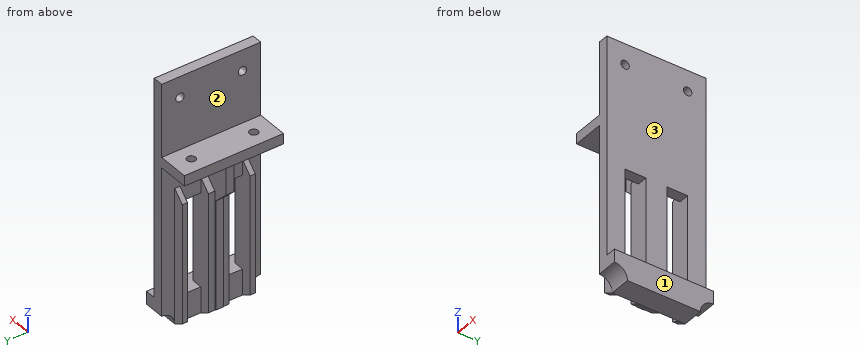
from build123d import *

# Parameters (mm, degrees)
F0_W      = 25.4
F0_H      = 228.6
F1_DEPTH  = 120.65
F2_DEPTH  = 76.2
F3_DEPTH  = 25.4
F4_R      = 10.31875
F5_DEPTH  = 101.601
F7_DEPTH  = 127.001
F9_DEPTH  = 88.9
F10_DEPTH = 76.2
F11_DEPTH = 25.4
F12_DEPTH = 9.525
F13_R     = 10.31875
F14_DEPTH = 419.031


with BuildPart() as f1:
    # F0 (on Front) → F1 (new body, symmetric)
    with BuildSketch(Plane.XZ):
        with Locations((-12.7, 114.3)):
            Rectangle(F0_W, F0_H)
        Polygon((-25.4, 228.6), (0, 228.6), (0, 533.6), (-25.4, 533.6), (-25.4, 355.73), (-101.6, 355.73), (-101.6, 330.33), (-25.4, 330.33), align=None)
        Polygon((25.4, 0), (0, 0), (-25.4, 0), (-25.4, -63.3), (25.4, -63.3), align=None)
    extrude(amount=F1_DEPTH, both=True)

    # F0 (on Front) → F2 (cut, symmetric)
    with BuildSketch(Plane.XZ):
        with Locations((-12.7, 114.3)):
            Rectangle(F0_W, F0_H)
    extrude(amount=F2_DEPTH, both=True, mode=Mode.SUBTRACT)

    # F0 (on Front) → F3 (join, symmetric)
    with BuildSketch(Plane.XZ):
        with Locations((-12.7, 114.3)):
            Rectangle(F0_W, F0_H)
    extrude(amount=F3_DEPTH, both=True)

    # F4 (on face) → F5 (cut, through all)
    with BuildSketch(Plane.YZ):
        with Locations((-76.2, 482.6)):
            Circle(F4_R)
        with Locations((76.2, 482.6)):
            Circle(F4_R)
    extrude(amount=-F5_DEPTH, mode=Mode.SUBTRACT)

    # F6 (on face) → F7 (cut, through all)
    with BuildSketch(Plane.YZ.offset(25.4)):
        with BuildLine():
            Line((-120.65, -63.3), (-88.9, -63.3))
            ThreePointArc((-88.9, -63.3), (-98.1993596973, -40.8493596973), (-120.65, -31.55))
            Line((-120.65, -31.55), (-120.65, -63.3))
        make_face()
        with BuildLine():
            ThreePointArc((120.65, -31.55), (98.1993596973, -40.8493596973), (88.9, -63.3))
            Line((88.9, -63.3), (120.65, -63.3))
            Line((120.65, -63.3), (120.65, -31.55))
        make_face()
    extrude(amount=-F7_DEPTH, mode=Mode.SUBTRACT)

    # F8 (on Front) → F9 (join, symmetric)
    with BuildSketch(Plane.XZ):
        Polygon((-50.8, -48.6353031626), (-25.4, -63.3), (-25.4, 266.83), (-50.8, 241.43), (-50.8, 216.03), align=None)
    extrude(amount=F9_DEPTH, both=True)

    # F8 (on Front) → F10 (cut, symmetric)
    with BuildSketch(Plane.XZ):
        Polygon((-50.8, -48.6353031626), (-25.4, -63.3), (-25.4, 266.83), (-50.8, 241.43), (-50.8, 216.03), align=None)
    extrude(amount=F10_DEPTH, both=True, mode=Mode.SUBTRACT)

    # F8 (on Front) → F11 (join, symmetric)
    with BuildSketch(Plane.XZ):
        Polygon((-50.8, -48.6353031626), (-25.4, -63.3), (-25.4, 266.83), (-50.8, 241.43), (-50.8, 216.03), align=None)
    extrude(amount=F11_DEPTH, both=True)

    # F8 (on Front) → F12 (join, symmetric)
    with BuildSketch(Plane.XZ):
        Polygon((-50.8, 241.43), (-25.4, 266.83), (-25.4, 330.33), (-88.9, 330.33), (-88.9, 254.13), (-53.975, 219.205), (-50.8, 216.03), align=None)
        Polygon((-53.975, -46.8022160579), (-50.8, -48.6353031626), (-50.8, 216.03), (-53.975, 219.205), align=None)
    extrude(amount=F12_DEPTH, both=True)

    # F13 (on face) → F14 (cut, through all)
    with BuildSketch(Plane.XY.offset(355.73)):
        with Locations((-63.5, 76.2)):
            Circle(F13_R)
        with Locations((-63.5, -76.2)):
            Circle(F13_R)
    extrude(amount=-F14_DEPTH, mode=Mode.SUBTRACT)


solid = f1.part
Could you check a few things on this model? Use its own coordinates, in mm. Face numbers are marked on the shaded views. A direction names the side the tool comes from. Round coordinates to 2 decimals unless told otherwise and drop trailing zeros. Write each loop counter-clockwise with the first axis right and the second up, starting at its lowest first coordinate (ties: lowest second). Pieces come first, ordered by that corner, then holes. Notation, with made-up numbers: (11.25, 54) - (44.25, 54) arc R24 cw to (44.25, 80) - close; hole circle Ø3 at (71, 5). An arc over 180 degrees is marked (long way). Use a Markdown table: item, result.
Q1. Please list where these lines run through material, in increasing order: L1, parallel to Y at x = -63, z = 343; L2, parallel to Y at x = -7.5, z = 203; L3, parallel to Z at x = -65, y = 105.
Output values:
| item | result |
|---|---|
| L1 | -120.65 to -86.51, -65.89 to 65.89, 86.51 to 120.65 |
| L2 | -120.65 to -76.2, -25.4 to 25.4, 76.2 to 120.65 |
| L3 | 330.33 to 355.73 |
Q2. For the marked faces 1, 2 and 3, which set-ups out of +Z, -Z, +X, -X, +Y, -Y let a thin tool reach every point of the face, with its end or its side?
Output values:
| item | result |
|---|---|
| face 1 | +Z, -Z, +X, +Y, -Y |
| face 2 | +Z, -X, +Y, -Y |
| face 3 | +Z, +X, +Y, -Y |
Q3. I want a section at D-D (z = 285). List the corners of the cut face in (x, y) for me (3 decimals), plus the area to 3 significant figures.
Output values:
| item | result |
|---|---|
| outline | (-88.9, -9.525) - (-25.4, -9.525) - (-25.4, -120.65) - (0, -120.65) - (0, 120.65) - (-25.4, 120.65) - (-25.4, 9.525) - (-88.9, 9.525) - close |
| area | 7,340 mm2 |
Q4. I want a section at A-A (z = 482.6). List the corners of the cut face in (x, y) for me, plus the area to 3 significant figures.
Output values:
| item | result |
|---|---|
| outline | (-25.4, -120.65) - (0, -120.65) - (0, -86.52) - (-25.4, -86.52) - close; (-25.4, -65.88) - (0, -65.88) - (0, 65.88) - (-25.4, 65.88) - close; (-25.4, 86.52) - (0, 86.52) - (0, 120.65) - (-25.4, 120.65) - close |
| area | 5,080 mm2 |
Q5. I want a section at B-B (x = -63.5). List the corners of the cut face in (y, z) for me (3 decimals), plus the area to 3 significant figures.
Output values:
| item | result |
|---|---|
| outline | (-120.65, 330.33) - (-86.519, 330.33) - (-86.519, 355.73) - (-120.65, 355.73) - close; (-65.881, 330.33) - (-9.525, 330.33) - (-9.525, 228.73) - (9.525, 228.73) - (9.525, 330.33) - (65.881, 330.33) - (65.881, 355.73) - (-65.881, 355.73) - close; (86.519, 330.33) - (120.65, 330.33) - (120.65, 355.73) - (86.519, 355.73) - close |
| area | 7,020 mm2 |
Q6. For pin 1 (1.5 mm diameter, centred on x = -48, y = -60, fed in from +Z); pin 2 (8 mm diameter, centred on y = -16, z = 52, fed in from -X); pin 3 (3 mm diameter, centred on x = 5, y = -74.5, fed in from +Z), each with a flat end and sliding along its axis, tell me the tip position at first contact or that it passes through.
Output values:
| item | result |
|---|---|
| pin 1 | z = 355.73 |
| pin 2 | x = -50.8 |
| pin 3 | z = 0 |
Q7. I want a section at C-C (y = -50). List the corners of the cut face in (x, z) for me.
Output values:
| item | result |
|---|---|
| outline | (-101.6, 330.33) - (-25.4, 330.33) - (-25.4, 228.6) - (0, 228.6) - (0, 533.6) - (-25.4, 533.6) - (-25.4, 355.73) - (-101.6, 355.73) - close; (-25.4, -63.3) - (25.4, -63.3) - (25.4, 0) - (-25.4, 0) - close |
